Input: part model. Units: mm. Frame: model coordinates. Face numbers are marked on the shaded views. Give positions to 0.01 mm unless a question says otherwise; leave off trailing zeros. Loops run counter-clockwise (first coordinate to the right, second up) from the corner with the lowest first, then second, coordinate; pieces in that order, holes last. Notation, with made-up numbers: (39.5, 52) -> (92.5, 52) arc R4 cw to (92.5, 59) -> close; hole circle Ø3 at (62, -13.75). An arc over 180 degrees is marked (long way). One line per question, with ' | ' between items.
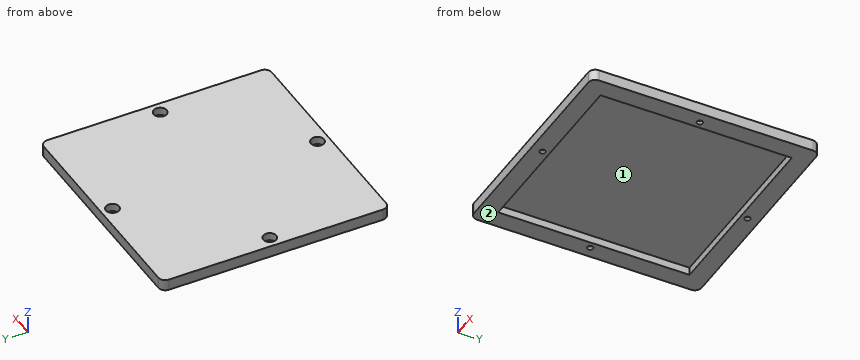
Autodesk Inventor part; units mm, degrees
ref_plane "YZ Plane" through (0, 0, 0) normal (1, 0, 0) x (0, 1, 0)
ref_plane "XZ Plane" through (0, 0, 0) normal (0, 1, 0) x (-1, 0, 0)
ref_plane "XY Plane" through (0, 0, 0) normal (0, 0, 1) x (1, 0, 0)
sketch "Sketch1" plane through (0, 0, 0) normal (0, 0, 1) x (1, 0, 0)
  line L0 (47, 50) -> (-47, 50)
  line L1 (-50, 47) -> (-50, -47)
  line L2 (-47, -50) -> (47, -50)
  line L3 (50, -47) -> (50, 47)
  line L4 (-48, 4) -> (-48, 48)
  line L5 (4, 48) -> (48, 48)
  line L6 (48, 48) -> (48, 4)
  line L7 (48, -48) -> (4, -48)
  arc A0 (47, -50) -> (50, -47) centre (47, -47) ccw
  arc A1 (50, 47) -> (47, 50) centre (47, 47) ccw
  arc A2 (-47, 50) -> (-50, 47) centre (-47, 47) ccw
  arc A3 (-50, -47) -> (-47, -50) centre (-47, -47) ccw
  circle A4 centre (0, -45) radius 1.25
  circle A5 centre (0, 45) radius 1.25
  circle A6 centre (-45, 0) radius 1.25
  circle A7 centre (45, 0) radius 1.25
  arc A8 (-43, -3) -> (-42, -2) centre (-43, -2) ccw
  line L8 (-42, -2) -> (-42, 2)
  arc A9 (-42, 2) -> (-43, 3) centre (-43, 2) ccw
  line L9 (-43, 3) -> (-47, 3)
  arc A10 (-48, 4) -> (-47, 3) centre (-47, 4) ccw
  arc A11 (-3, 47) -> (-4, 48) centre (-4, 47) ccw
  line L10 (-3, 47) -> (-3, 43)
  arc A12 (-3, 43) -> (-2, 42) centre (-2, 43) ccw
  line L11 (-2, 42) -> (2, 42)
  arc A13 (2, 42) -> (3, 43) centre (2, 43) ccw
  line L12 (3, 43) -> (3, 47)
  arc A14 (4, 48) -> (3, 47) centre (4, 47) ccw
  arc A15 (47, 3) -> (48, 4) centre (47, 4) ccw
  line L13 (47, 3) -> (43, 3)
  arc A16 (43, 3) -> (42, 2) centre (43, 2) ccw
  line L14 (42, 2) -> (42, -2)
  arc A17 (42, -2) -> (43, -3) centre (43, -2) ccw
  line L15 (43, -3) -> (47, -3)
  arc A18 (48, -4) -> (47, -3) centre (47, -4) ccw
  arc A19 (3, -47) -> (4, -48) centre (4, -47) ccw
  line L16 (3, -47) -> (3, -43)
  arc A20 (3, -43) -> (2, -42) centre (2, -43) ccw
  line L17 (2, -42) -> (-2, -42)
  arc A21 (-2, -42) -> (-3, -43) centre (-2, -43) ccw
  line L18 (-3, -43) -> (-3, -47)
  arc A22 (-4, -48) -> (-3, -47) centre (-4, -47) ccw
  arc A23 (-47, -3) -> (-48, -4) centre (-47, -4) ccw
  line L19 (-47, -3) -> (-43, -3)
  line L20 (-48, 48) -> (-4, 48)
  line L21 (48, -4) -> (48, -48)
  line L22 (-4, -48) -> (-48, -48)
  line L23 (-48, -48) -> (-48, -4)
  point P0 (0, 0)
  point P1 (-47, 4)
  point P2 (-4, 47)
  point P3 (4, 47)
  point P4 (47, 4)
  point P5 (47, -4)
  point P6 (4, -47)
  point P7 (-4, -47)
  point P8 (-47, -4)
extrude "Extrusion1" add sketch "Sketch1" along normal blind 5 contours A1 L3 A0 L2 A3 L1 A2 L0 | L4 L20 A11 L10 A12 L11 A13 L12 A14 L5 L6 A15 L13 A16 L14 A17 L15 A18 L21 L7 A19 L16 A20 L17 A21 L18 A22 L22 L23 A23 L19 A8 L8 A9 L9 A10
sketch "Sketch2" plane through (0, 0, 5) normal (0, 0, 1) x (1, 0, 0)
  circle A0 centre (45, 0) radius 1.25
  circle A1 centre (45, 0) radius 2.875
  circle A2 centre (0, 45) radius 2.875
  circle A3 centre (-45, 0) radius 2.875
  circle A4 centre (0, -45) radius 2.875
  point P0 (0, 0)
  dimension "d2" = 5.75
  dimension "d5" = 360
extrude "Extrusion2" cut sketch "Sketch2" against normal blind 3.5 contours A0 | A1 | A2 | A3 | A4
sketch "Sketch3" plane through (0, 0, 0) normal (0, 0, -1) x (-1, 0, 0)
  line L0 (-42, 42) -> (42, 42)
  line L1 (42, 42) -> (42, -42)
  line L2 (42, -42) -> (-42, -42)
  line L3 (-42, -42) -> (-42, 42)
  line L4 (-42, 42) -> (42, -42) construction
  line L5 (42, 42) -> (-42, -42) construction
  point P0 (0, 0)
  dimension "d9" = 84
  dimension "d10" = 84
extrude "Extrusion3" cut sketch "Sketch3" against normal blind 3.5
properties part number "BaseBottom"
1. Pull-direction query (Y, two-part tool) for the marked faces 1 and 2; classes: pulls with the +Y half, pulls with the -Y half, needs draft (parallel to the pull), parting line crosses it, or undercut.
Determined:
face 1: undercut | face 2: needs draft
2. Ray query, line 1 along X through (y, z) = (-45, 1.15); line 2 along X through (y, z) = (18.5, 0.75); line 3 along Y through (x, z) = (-45, 3) (3 decimals). Return the intervals inside material, ascending. Write a range as from..to.
Determined:
line 1: x = -50..-1.25, 1.25..50 | line 2: x = -50..-42, 42..50 | line 3: y = -50..-2.875, 2.875..50
3. Section query A-A (y = -45). Output: boundary loops of the cut face in (x, z) (3 decimals).
Determined:
outline: (-50, 0) -> (-1.25, 0) -> (-1.25, 1.5) -> (-2.875, 1.5) -> (-2.875, 5) -> (-50, 5) -> close; (1.25, 0) -> (50, 0) -> (50, 5) -> (2.875, 5) -> (2.875, 1.5) -> (1.25, 1.5) -> close
4. Pin query (flat end, axial travel): P1, Ø1.5, axis at x = 45, y = 0, coming from the +Z side; P2, Ø12, axis at x = 23, y = -12.5, coming from the -Z side. Return the tip coordinate at first contact, or that it passes through.
Determined:
P1: passes through | P2: stops at z = 3.5
5. Section query B-B (x = 0). Output: boundary loops of the cut face in (y, z) (3 decimals).
Determined:
outline: (-50, 0) -> (-46.25, 0) -> (-46.25, 1.5) -> (-47.875, 1.5) -> (-47.875, 5) -> (-50, 5) -> close; (-43.75, 0) -> (-42, 0) -> (-42, 3.5) -> (42, 3.5) -> (42, 0) -> (43.75, 0) -> (43.75, 1.5) -> (42.125, 1.5) -> (42.125, 5) -> (-42.125, 5) -> (-42.125, 1.5) -> (-43.75, 1.5) -> close; (46.25, 0) -> (50, 0) -> (50, 5) -> (47.875, 5) -> (47.875, 1.5) -> (46.25, 1.5) -> close
